Part model, mm, in its own coordinate system. Give positions to 0.01 mm unless a question says otherwise; leave off trailing zeros. Loops run counter-clockwise (first coordinate to the right, second up) from the corner with the lowest first, then second, coordinate; pieces in that order, holes last. Notation, with made-up numbers: M -39.75,-12 L -34.75,-12 A15 ccw -34.75,9 Z; hole C 78,50.25 d11. An arc over 180 degrees is marked long. Answer in a Markdown table with one row per item.
Autodesk Inventor part; units mm, degrees
ref_plane "YZ Plane" through (0, 0, 0) normal (1, 0, 0) x (0, 1, 0)
ref_plane "XZ Plane" through (0, 0, 0) normal (0, 1, 0) x (-1, 0, 0)
ref_plane "XY Plane" through (0, 0, 0) normal (0, 0, 1) x (1, 0, 0)
sketch "Sketch1" plane through (0, 0, 0) normal (0, 0, 1) x (1, 0, 0)
  line L0 (-15.6535, 8.2698) -> (22.4465, 8.2698)
  line L1 (22.4465, 8.2698) -> (22.4465, -10.7802)
  line L2 (22.4465, -10.7802) -> (-15.6535, -10.7802)
  line L3 (-15.6535, -10.7802) -> (-15.6535, 8.2698)
  circle A0 centre (3.3965, -1.2552) radius 3
  point P0 (0, 0)
  dimension "d0" = 38.1
  dimension "d1" = 19.05
  dimension "d4" = 6
extrude "Extrusion1" add sketch "Sketch1" along normal blind 3.175 contours L0 L1 L2 L3 | A0
extrude "Extrusion2" cut sketch "Sketch1" along normal blind 3.175 contours A0
properties part number "CURM_Caterpillar_Tail"
(1) Saw through at B-B (z = 2.25). Write the cut outline in (x, y), plus the area to 3 significant figures.
Recorded:
| item | result |
|---|---|
| outline | M -15.65,-10.78 L 22.45,-10.78 L 22.45,8.27 L -15.65,8.27 Z; hole C 3.4,-1.26 d6 |
| area | 698 mm^2 |
(2) Pull direction Y, two halves, no side cores. Call faces 1 (the face through (4, -10.78, 2)), 2 (the face through (22.446, -1, 2)), 3 (the face through (1.2, -3.3, 1.6)): +Y half, -Y half, draft (parallel to the pull), parting line (faces both ways), or undercut.
Recorded:
| item | result |
|---|---|
| face 1 | -Y half |
| face 2 | draft |
| face 3 | undercut |
(3) Drill centre lines: line 1 along X through (y, z) = (0, 2.45); line 2 along Y through (x, z) = (1, 0.45); line 3 along Y through (x, z) = (1.5, 1.9). Where is each one in solid material? Low to high.
Recorded:
| item | result |
|---|---|
| line 1 | x = -15.65 to 0.67, 6.12 to 22.45 |
| line 2 | y = -10.78 to -3.06, 0.55 to 8.27 |
| line 3 | y = -10.78 to -3.58, 1.07 to 8.27 |
(4) Pin check, flat tip, straight feed: pin 1 Ø5 at (x, y) = (3.4, -1.26) entering from -Z. Stop position of the tip, or through.
Recorded:
| item | result |
|---|---|
| pin 1 | passes through |
(5) Saw through at A-A (y = 0.25). Write the cut outline in (x, z) (1 decimal), plus the area to 3 significant figures.
Recorded:
| item | result |
|---|---|
| outline | M -15.7,0 L 0.8,0 L 0.8,3.2 L -15.7,3.2 Z; M 6,0 L 22.4,0 L 22.4,3.2 L 6,3.2 Z |
| area | 104 mm^2 |
(6) Saw through at C-C (y = -3). Write the cut outline in (x, z) (1 decimal).
Recorded:
| item | result |
|---|---|
| outline | M -15.7,0 L 1,0 L 1,3.2 L -15.7,3.2 Z; M 5.8,0 L 22.4,0 L 22.4,3.2 L 5.8,3.2 Z |
